```python
from build123d import *

# Parameters (mm, degrees)
SKETCH1_W           = 152.0063
SKETCH1_H           = 38.01618
SKETCH1_W_2         = 146.17954
SKETCH1_H_2         = 32.18942
BOSS_EXTRUDE1_DEPTH = 101.6
CUT_EXTRUDE1_START  = 16.09471
SKETCH2_R           = 12.578868564
SKETCH2_R_2         = 3.175
CUT_EXTRUDE1_DEPTH  = 2.91338
SKETCH3_R           = 3.175
CUT_EXTRUDE2_DEPTH  = 2.91338


with BuildPart() as part:
    # Sketch1 → Boss-Extrude1 (new, symmetric)
    with BuildSketch(Plane.XY):
        Rectangle(SKETCH1_W, SKETCH1_H)
        Rectangle(SKETCH1_W_2, SKETCH1_H_2, mode=Mode.SUBTRACT)
    extrude(amount=BOSS_EXTRUDE1_DEPTH, both=True)

    # Sketch2 (on Top Plane) → Cut-Extrude1 (cut)
    with BuildSketch(Plane(origin=(0, 0, 0), x_dir=(1, 0, 0), z_dir=(0, 1, 0)).offset(CUT_EXTRUDE1_START)):
        with Locations(Location((-50.60315, -76.2, 0), (0, 0, 270))):
            Circle(SKETCH2_R)
        with Locations(Location((-50.60315, -44.45, 0), (0, 0, 270))):
            Circle(SKETCH2_R)
        with Locations(Location((-50.60315, 76.2, 0), (0, 0, 270))):
            Circle(SKETCH2_R_2)
        with Locations(Location((-50.60315, 50.8, 0), (0, 0, 270))):
            Circle(SKETCH2_R_2)
        with Locations(Location((-50.60315, 25.4, 0), (0, 0, 270))):
            Circle(SKETCH2_R_2)
        with Locations(Location((-50.60315, 0, 0), (0, 0, 270))):
            Circle(SKETCH2_R_2)
        with Locations(Location((-25.20315, 76.2, 0), (0, 0, 270))):
            Circle(SKETCH2_R_2)
        with Locations(Location((-25.20315, 50.8, 0), (0, 0, 270))):
            Circle(SKETCH2_R_2)
        with Locations(Location((-25.20315, 25.4, 0), (0, 0, 270))):
            Circle(SKETCH2_R_2)
        with Locations(Location((-25.20315, 0, 0), (0, 0, 270))):
            Circle(SKETCH2_R_2)
    extrude(amount=CUT_EXTRUDE1_DEPTH, mode=Mode.SUBTRACT)

    # Sketch3 → Cut-Extrude2 (cut)
    with BuildSketch(Plane(origin=(76.00315, 0, 0), x_dir=(0, 0, -1), z_dir=(1, 0, 0))):
        with Locations((-12.7, 6.30809)):
            Circle(SKETCH3_R)
        with Locations((12.7, 6.30809)):
            Circle(SKETCH3_R)
        with Locations((38.1, 6.30809)):
            Circle(SKETCH3_R)
        with Locations((63.5, 6.30809)):
            Circle(SKETCH3_R)
        with Locations((88.9, 6.30809)):
            Circle(SKETCH3_R)
        with Locations((88.9, -6.30809)):
            Circle(SKETCH3_R)
        with Locations((63.5, -6.30809)):
            Circle(SKETCH3_R)
        with Locations((38.1, -6.30809)):
            Circle(SKETCH3_R)
        with Locations((12.7, -6.30809)):
            Circle(SKETCH3_R)
        with Locations((-12.7, -6.30809)):
            Circle(SKETCH3_R)
        with Locations((-38.1, -6.30809)):
            Circle(SKETCH3_R)
        with Locations((-63.5, -6.30809)):
            Circle(SKETCH3_R)
        with Locations((-88.9, -6.30809)):
            Circle(SKETCH3_R)
        with Locations((-88.9, 6.30809)):
            Circle(SKETCH3_R)
        with Locations((-63.5, 6.30809)):
            Circle(SKETCH3_R)
        with Locations((-38.1, 6.30809)):
            Circle(SKETCH3_R)
    extrude(amount=-CUT_EXTRUDE2_DEPTH, mode=Mode.SUBTRACT)


solid = part.part
```
Can you work these out from the model? Positions are in its coordinate system, mm. A direction names the side the tool comes from. Coordinates: 2 decimals unless noted, no trailing zeros. Loops run counter-clockwise (first coordinate to the right, second up) from the corner with the lowest first, then second, coordinate; pieces in that order, holes last. Notation, with made-up numbers: (-16.75, 62.25) -> (-6.75, 62.25) arc R19 ccw to (-6.75, 71.25) -> close; hole circle Ø9 at (-36.5, 46.5). An arc over 180 degrees is marked (long way). Put each result on its own line as item: value. Start each with the question number.
Q1. I want a section at D-D (z = 76.2). Write out the boundary of the cut face in (x, y), plus the area to 4 significant figures.
Q2. I want a section at A-A (x = 18.5). Write out the boundary of the cut face in (y, z), plus the area to 3 significant figures.
Q3. If I drill on line 1 (Y direction, x = 73.8, z = 88.9); line 2 (Y direction, x = 47.5, z = 82.5); line 3 (X direction, y = 4, z = -3), over which ranges is the centre line in solid material (lowest first)? Write a range as [from, to].
Q4. For faces 4 (the face through (-1, 19.008, 1)), 5 (the face through (-73.09, 0, 1)), 6 (the face through (-28, 17.5, -74.7)), 7 (the face through (74.57, 6.45, -34.93)), 8 (the face through (-12, -17, -101.6)), which set-ups out of +Z, -Z, +X, -X, +Y, -Y let a thin tool reach every point of the face, with its end or its side?
Q5. I want a section at B-B (y = -13.5). Write out the boundary of the cut face in (x, z), plus the area to 3 significant figures.
Q6. Thinking about a two-plate mould opening in Z: for faces 1 (the face through (-1, -19.008, 1)), 2 (the face through (-51.819, 17.531, -22.467)), 3 (the face through (-12, -17, 101.6)), which applies, pulls with the +Z half, pulls with the -Z half, needs draft (parallel to the pull), parting line crosses it, or undercut?
Q7. I want a section at C-C (z = -25.4). Write out the boundary of the cut face in (x, y), plus the area to 3 significant figures.
Q8. I'm going to push a flat-ended pin straight in: P1, Ø5.5, axis at x = -25.2, z = 0, coming from the +Y side. Where does the tip first touch, or does it pass through?
Taken from the geometry:
1. outline: (-76, -19.01) -> (76, -19.01) -> (76, 19.01) -> (-38.02, 19.01) -> (-38.02, 16.09) -> (73.09, 16.09) -> (73.09, -16.09) -> (-73.09, -16.09) -> (-73.09, 16.09) -> (-63.18, 16.09) -> (-63.18, 19.01) -> (-76, 19.01) -> close
1. area: 1,000 mm2
2. outline: (-19.01, -101.6) -> (-16.09, -101.6) -> (-16.09, 101.6) -> (-19.01, 101.6) -> close; (16.09, -101.6) -> (19.01, -101.6) -> (19.01, 101.6) -> (16.09, 101.6) -> close
2. area: 1,180 mm2
3. line 1: y = [-19.01, -9.48], [-3.13, 3.13], [9.48, 19.01]
3. line 2: y = [-19.01, -16.09], [16.09, 19.01]
3. line 3: x = [-76, -73.09], [73.09, 76]
4. face 4: +Z, -Z, +X, -X, +Y
4. face 5: +Z, -Z
4. face 6: +Y
4. face 7: +X
4. face 8: -Z, +X, -X, +Y, -Y
5. outline: (-76, -101.6) -> (-73.09, -101.6) -> (-73.09, 101.6) -> (-76, 101.6) -> close; (73.09, -101.6) -> (76, -101.6) -> (76, 101.6) -> (73.09, 101.6) -> close
5. area: 1,180 mm2
6. face 1: needs draft
6. face 2: undercut
6. face 3: pulls with the +Z half
7. outline: (-76, -19.01) -> (76, -19.01) -> (76, 19.01) -> (-22.03, 19.01) -> (-22.03, 16.09) -> (73.09, 16.09) -> (73.09, -16.09) -> (-73.09, -16.09) -> (-73.09, 16.09) -> (-53.78, 16.09) -> (-53.78, 19.01) -> (-76, 19.01) -> close; (-47.43, 16.09) -> (-28.38, 16.09) -> (-28.38, 19.01) -> (-47.43, 19.01) -> close
7. area: 1,040 mm2
8. P1: stops at y = -16.09
